Source: CAD feature listing. Evaluate the final solid. Frame: model axes, mm. Face numbers are marked on the shaded views. A direction names the side the tool comes from. Coordinates: 2 decimals unless noted, no trailing zeros. Write each loop counter-clockwise with the first axis right and the second up, starting at its lowest first coordinate (ties: lowest second). Pieces come first, ordered by that corner, then holes. Notation, with made-up numbers: M 53,10 L 80,10 A9 ccw 80,21 Z; hole C 9,89.5 d8. An arc over 180 degrees is marked long. One line per item, written item: value. Start each with the question number.
Item 1: Cut plane B-B, the plane x = 58.96. State how many separate pieces and enclosed holes the cut face has, then the cut area to 3 significant figures.
Item 2: Pin query (flat end, axial travel): P1, Ø1.6, axis at x = 5, z = 64.5, coming from the +Y side; P2, Ø19, axis at x = 87.5, z = 35, coming from the +Y side; P3, Ø1.5, axis at x = 92.5, z = 57.5, coming from the +Y side; P4, Ø6, axis at x = 59, z = 20.5, coming from the -Y side. Return the tip coordinate at first contact, or that it passes through.
Item 3: Ray query, L1, parallel to X at y = 83.75, z = 5; L2, parallel to Z at x = 130, y = 91; L3, parallel to X at y = 91, z = 65. Return the intervals inside material, ascending. Write a range as from..to.
Item 4: Cut plane C-C, the plane y = 35. Output: boundary loops of the cut face in (x, z), then the cut area to 3 significant figures.
Item 5: Cut plane A-A, the plane y = 56. Output: boundary loops of the cut face in (x, z), then the cut area to 3 significant figures.
Item 6: Set-up query: the marked faces 1 and 2. Return all of +Z, -Z, +X, -X, +Y, -Y with unobstructed straight access to the full face (end or side cutting, diameter ignored); none if empty.
```python
from build123d import *

# Parameters (mm, degrees)
SKETCH1_W           = 135
SKETCH1_H           = 70
BOSS_EXTRUDE1_DEPTH = 96
SKETCH10_W          = 115
SKETCH10_H          = 50
CUT_EXTRUDE7_DEPTH  = 91
SKETCH2_R           = 2.25
CUT_EXTRUDE1_DEPTH  = 178.217380637
SKETCH3_R           = 5
CUT_EXTRUDE2_DEPTH  = 178.217380637
SKETCH6_R           = 2
CUT_EXTRUDE5_DEPTH  = 7.4
CUT_EXTRUDE9_REACH  = 188.188
SKETCH17_R          = 8
SKETCH19_R          = 1
CUT_EXTRUDE12_DEPTH = 20
SKETCH23_R          = 12
CUT_EXTRUDE13_DEPTH = 7
SKETCH7_R           = 8.25
SKETCH7_R_2         = 5
CUT_EXTRUDE14_DEPTH = 4.5
SKETCH24_R          = 3.25
CUT_EXTRUDE15_DEPTH = 2
FILLET1_R           = 3
BOSS_EXTRUDE2_DEPTH = 3
FILLET2_R           = 0.5


with BuildPart() as part:
    # Sketch1 → Boss-Extrude1 (new body)
    with BuildSketch(Plane(origin=(0, 0, 0), x_dir=(1, 0, 0), z_dir=(0, 1, 0))):
        with Locations((67.5, -35)):
            Rectangle(SKETCH1_W, SKETCH1_H)
    extrude(amount=BOSS_EXTRUDE1_DEPTH)

    # Sketch10 → Cut-Extrude7 (cut)
    with BuildSketch(Plane(origin=(0, 96, 0), x_dir=(1, 0, 0), z_dir=(0, 1, 0))):
        with Locations((67.5, -35)):
            Rectangle(SKETCH10_W, SKETCH10_H)
    extrude(amount=-CUT_EXTRUDE7_DEPTH, mode=Mode.SUBTRACT)

    # Sketch2 → Cut-Extrude1 (cut, through all)
    with BuildSketch(Plane(origin=(0, 5, 0), x_dir=(1, 0, 0), z_dir=(0, 1, 0))):
        with Locations(Location((58.96, -21, 0), (0, 0, 270))):
            Circle(SKETCH2_R)
        with Locations(Location((98.96, -21, 0), (0, 0, 270))):
            Circle(SKETCH2_R)
        with Locations(Location((58.96, -49, 0), (0, 0, 270))):
            Circle(SKETCH2_R)
        with Locations(Location((98.96, -49, 0), (0, 0, 270))):
            Circle(SKETCH2_R)
    extrude(amount=-CUT_EXTRUDE1_DEPTH, mode=Mode.SUBTRACT)

    # Sketch3 → Cut-Extrude2 (cut, through all)
    with BuildSketch(Plane(origin=(0, 5, 0), x_dir=(1, 0, 0), z_dir=(0, 1, 0))):
        with Locations(Location((87.5, -35, 0), (0, 0, 270))):
            Circle(SKETCH3_R)
    extrude(amount=-CUT_EXTRUDE2_DEPTH, mode=Mode.SUBTRACT)

    # Sketch6 → Cut-Extrude5 (cut)
    with BuildSketch(Plane(origin=(0, 96, 0), x_dir=(1, 0, 0), z_dir=(0, 1, 0))):
        with Locations(Location((130, -65, 0), (0, 0, 270))):
            Circle(SKETCH6_R)
        with Locations(Location((5, -65, 0), (0, 0, 270))):
            Circle(SKETCH6_R)
        with Locations(Location((5, -5, 0), (0, 0, 270))):
            Circle(SKETCH6_R)
        with Locations(Location((130, -5, 0), (0, 0, 270))):
            Circle(SKETCH6_R)
    extrude(amount=-CUT_EXTRUDE5_DEPTH, mode=Mode.SUBTRACT)

    # Sketch17 → Cut-Extrude9 (cut, up to next)
    with BuildSketch(Plane(origin=(0, 0, 85), x_dir=(0, 0, -1), z_dir=(1, 0, 0)), mode=Mode.PRIVATE) as cut_extrude9_sk1:
        with Locations(Location((50, 56, 0), (0, 0, 180))):
            Circle(SKETCH17_R)
    cut_extrude9_tool1 = extrude(cut_extrude9_sk1.sketch, amount=CUT_EXTRUDE9_REACH, mode=Mode.PRIVATE) & part.part
    add(cut_extrude9_tool1.solids().sort_by_distance((0, 56, 35))[0], mode=Mode.SUBTRACT)

    # Sketch19 → Cut-Extrude12 (cut)
    with BuildSketch(Plane(origin=(0, 88.6, 0), x_dir=(1, 0, 0), z_dir=(0, 1, 0))):
        with Locations(Location((5, -5, 0), (0, 0, 270))):
            Circle(SKETCH19_R)
        with Locations(Location((130, -5, 0), (0, 0, 270))):
            Circle(SKETCH19_R)
        with Locations(Location((130, -65, 0), (0, 0, 270))):
            Circle(SKETCH19_R)
        with Locations(Location((5, -65, 0), (0, 0, 270))):
            Circle(SKETCH19_R)
    extrude(amount=-CUT_EXTRUDE12_DEPTH, mode=Mode.SUBTRACT)

    # Sketch23 → Cut-Extrude13 (cut)
    with BuildSketch(Plane(origin=(10, 0, 0), x_dir=(0, 0, -1), z_dir=(1, 0, 0))):
        with Locations((-35, 56)):
            Circle(SKETCH23_R)
    extrude(amount=-CUT_EXTRUDE13_DEPTH, mode=Mode.SUBTRACT)

    # Sketch7 → Cut-Extrude14 (cut)
    with BuildSketch(Plane(origin=(0, 5, 0), x_dir=(1, 0, 0), z_dir=(0, 1, 0))):
        with Locations(Location((87.5, -35, 0), (0, 0, 270))):
            Circle(SKETCH7_R)
        with Locations(Location((87.5, -35, 0), (0, 0, 270))):
            Circle(SKETCH7_R_2, mode=Mode.SUBTRACT)
    extrude(amount=-CUT_EXTRUDE14_DEPTH, mode=Mode.SUBTRACT)

    # Sketch24 → Cut-Extrude15 (cut)
    with BuildSketch(Plane(origin=(0, 5, 0), x_dir=(1, 0, 0), z_dir=(0, 1, 0))):
        with Locations(Location((58.96, -21, 0), (0, 0, 270))):
            Circle(SKETCH24_R)
        with Locations(Location((98.96, -21, 0), (0, 0, 270))):
            Circle(SKETCH24_R)
        with Locations(Location((58.96, -49, 0), (0, 0, 270))):
            Circle(SKETCH24_R)
        with Locations(Location((98.96, -49, 0), (0, 0, 270))):
            Circle(SKETCH24_R)
    extrude(amount=-CUT_EXTRUDE15_DEPTH, mode=Mode.SUBTRACT)

    # Fillet1
    fillet1_edges = [part.edges().sort_by_distance(p)[0] for p in [
        (67.5, 5, 10),
        (10, 50.5, 10),
        (125, 5, 35),
        (125, 50.5, 10),
        (67.5, 5, 60),
        (125, 50.5, 60),
        (10, 5, 35),
        (10, 50.5, 60),
        (67.5, 0, 0),
        (135, 0, 35),
        (67.5, 0, 70),
        (0, 0, 35),
        (0, 48, 0),
        (135, 48, 0),
        (135, 48, 70),
        (0, 48, 70),
    ]]
    fillet(fillet1_edges, radius=FILLET1_R)

    # Sketch25 → Boss-Extrude2 (add)
    with BuildSketch(Plane(origin=(0, 96, 0), x_dir=(1, 0, 0), z_dir=(0, 1, 0))):
        with BuildLine():
            Line((128, -57), (128, -13))
            ThreePointArc((128, -13), (126.242640687, -8.757359313), (122, -7))
            Line((122, -7), (13, -7))
            ThreePointArc((13, -7), (8.757359313, -8.757359313), (7, -13))
            Line((7, -13), (7, -57))
            ThreePointArc((7, -57), (8.757359313, -61.242640687), (13, -63))
            Line((13, -63), (122, -63))
            ThreePointArc((122, -63), (126.242640687, -61.242640687), (128, -57))
        make_face()
        with BuildLine():
            Line((125, -13), (125, -57))
            ThreePointArc((125, -57), (124.121320344, -59.121320344), (122, -60))
            Line((122, -60), (13, -60))
            ThreePointArc((13, -60), (10.878679656, -59.121320344), (10, -57))
            Line((10, -57), (10, -13))
            ThreePointArc((10, -13), (10.878679656, -10.878679656), (13, -10))
            Line((13, -10), (122, -10))
            ThreePointArc((122, -10), (124.121320344, -10.878679656), (125, -13))
        make_face(mode=Mode.SUBTRACT)
    extrude(amount=BOSS_EXTRUDE2_DEPTH)

    # Fillet2
    fillet2_edges = [part.edges().sort_by_distance(p)[0] for p in [
        (126.242640687, 99, 61.242640687),
        (128, 99, 35),
        (126.242640687, 99, 8.757359313),
        (67.5, 99, 7),
        (8.757359313, 99, 8.757359313),
        (7, 99, 35),
        (8.757359313, 99, 61.242640687),
        (67.5, 99, 63),
        (124.121320344, 99, 10.878679656),
        (67.5, 99, 10),
        (10.878679656, 99, 10.878679656),
        (10, 99, 35),
        (10.878679656, 99, 59.121320344),
        (67.5, 99, 60),
        (124.121320344, 99, 59.121320344),
        (125, 99, 35),
    ]]
    fillet(fillet2_edges, radius=FILLET2_R)


solid = part.part
```
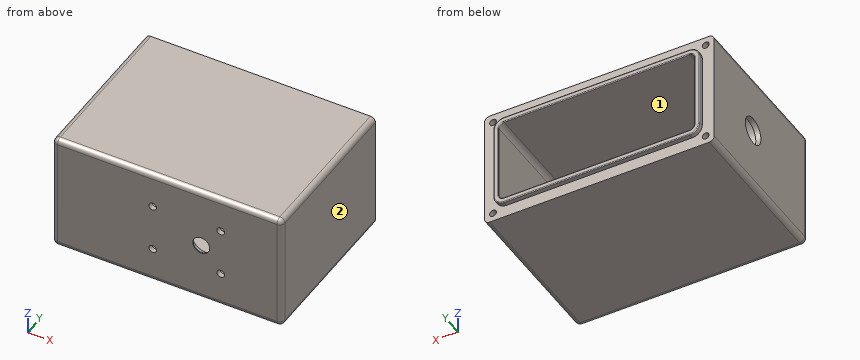
From the geometry:
1. separate pieces: 3
1. enclosed holes: 0
1. area: 2,130 mm²
2. P1: stops at y = 88.6
2. P2: stops at y = 5
2. P3: stops at y = 5.27
2. P4: stops at y = 0
3. L1: x = 0..4, 6..129, 131..135
3. L2: z = 0..3, 7..63, 67..70
3. L3: x = 0..3, 7..128, 132..135
4. outline: M 0,3 A3 ccw 3,0 L 132,0 A3 ccw 135,3 L 135,67 A3 ccw 132,70 L 3,70 A3 ccw 0,67 Z; hole M 10,13 A3 ccw 13,10 L 122,10 A3 ccw 125,13 L 125,57 A3 ccw 122,60 L 13,60 A3 ccw 10,57 Z
4. area: 3,700 mm²
5. outline: M 0,3 A3 ccw 3,0 L 132,0 A3 ccw 135,3 L 135,67 A3 ccw 132,70 L 3,70 A3 ccw 0,67 L 0,43 L 3,43 L 3,47 L 10,47 L 10,57 A3 cw 13,60 L 122,60 A3 cw 125,57 L 125,13 A3 cw 122,10 L 13,10 A3 cw 10,13 L 10,23 L 3,23 L 3,27 L 0,27 Z
5. area: 3,480 mm²
6. face 1: +Y
6. face 2: +Z, -Z, +X, +Y, -Y
